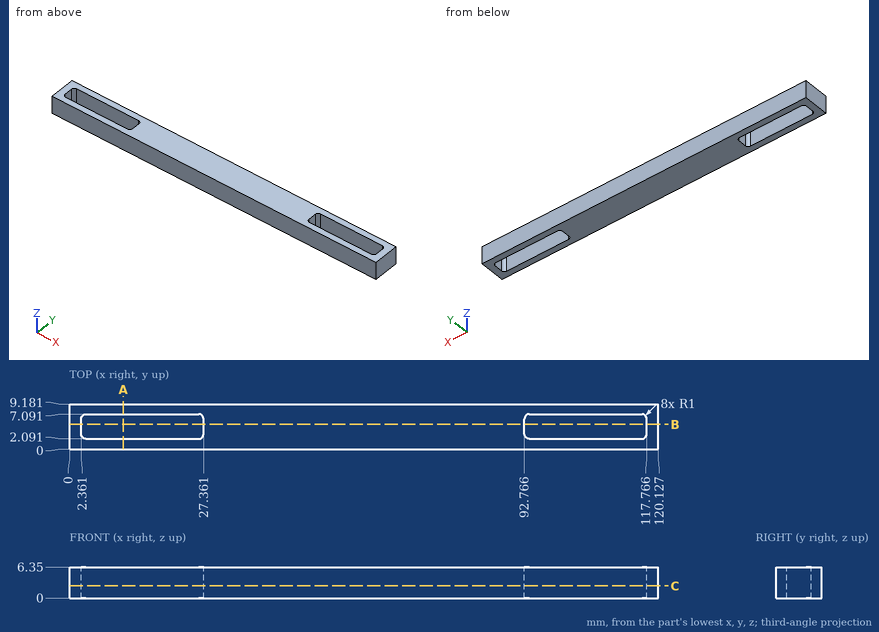
Job drawing, mm, ordinate dimensions from the low corner. One solid piece. Give positions to 0.01 mm unless a question says otherwise; leave off trailing zeros. Loops run counter-clockwise (first coordinate to the right, second up) from the corner with the lowest first, then second, coordinate; pieces in that order, holes last.
Item 1: Slice it at A-A, the plane x = 11. List the corners of the cut face in (y, z).
Answers follow:
outline: (0, 0) - (2.09, 0) - (2.09, 6.35) - (0, 6.35) - close; (7.09, 0) - (9.18, 0) - (9.18, 6.35) - (7.09, 6.35) - close
Item 2: Drill centre lines: line 1 (X direction, y = 5.25, z = 4.5) (1 decimal); line 2 (Y direction, x = 5, z = 2.75); line 3 (X direction, y = 2.5, z = 5.5) (1 decimal). Where is each one in solid material? Low to high.
Answers follow:
line 1: x = 0 to 2.4, 27.4 to 92.8, 117.8 to 120.1
line 2: y = 0 to 2.09, 7.09 to 9.18
line 3: x = 0 to 2.6, 27.2 to 93, 117.6 to 120.1
Item 3: Slice it at B-B, the plane y = 5. Give the number of separate pieces and of enclosed holes in the cut face, and give its area (3 significant figures).
Answers follow:
separate pieces: 3
enclosed holes: 0
area: 445 mm2
Item 4: Flat gauge pin, fed straight in: pin 1 (1.9 mm diameter, centred on x = 10, z = 4, fed in from -Y). Where does the tip first touch, or does it go through?
Answers follow:
pin 1: stops at y = 0
Item 5: Slice it at C-C, the plane z = 2.5. List the corners of the cut face in (x, y) (1 decimal).
Answers follow:
outline: (0, 0) - (120.1, 0) - (120.1, 9.2) - (0, 9.2) - close; hole (2.4, 3.1) arc R1 ccw to (3.4, 2.1) - (26.4, 2.1) arc R1 ccw to (27.4, 3.1) - (27.4, 6.1) arc R1 ccw to (26.4, 7.1) - (3.4, 7.1) arc R1 ccw to (2.4, 6.1) - close; hole (92.8, 3.1) arc R1 ccw to (93.8, 2.1) - (116.8, 2.1) arc R1 ccw to (117.8, 3.1) - (117.8, 6.1) arc R1 ccw to (116.8, 7.1) - (93.8, 7.1) arc R1 ccw to (92.8, 6.1) - close
